For this review, use the dimensioned drawing (mm, ordinates from the lowest corner) and the shaded views. A direction names the side the tool comes from. Coordinates: 2 decimals unless noted, no trailing zeros. Loops run counter-clockwise (first coordinate to the right, second up) from the corner with the lowest first, then second, coordinate; pieces in that order, holes last. Notation, with made-up numbers: (-13, -31) - (30, -31) arc R31 ccw to (30, -4) - close; hole circle Ø2 at (-7.75, 10.5). An arc over 180 degrees is marked (long way). Answer in a Markdown table with one row per item. Add a question column.
(1) The part is to be moulded in two halves that separate along X. For the marked faces 4, 5 and 6, say which applies: released by +X, released by -X, zero draft, split by the parting line, or undercut.
(2) For the marked faces 1, 2 and 3, list the 3-axis set-ups (+Z, -Z, +X, -X, +Y, -Y) from which the entire face can be reached by the end or side of a thin tool; tool diameter is ignored.
(3) Clearance check with flat-ended pins moving along their axes: pin 1 (5 mm diameter, centred on x = 12.5, y = 2, fed in from -Z); pin 2 (6 mm diameter, centred on x = 7, y = 3, fed in from +Z). State where each tip first meets the part, or that it passes through.
(4) We need section A-A, the plane z = 102. Write out the cut boundary in (x, y), plus the area to 3 significant figures.
(5) To check wall thickness, follow L1, parallel to X at y = 9.25, z = 40; L2, parallel to Z at x = 9.75, y = 9.5; L3, parallel to Z at x = 17.5, y = 8.75. State the ranges of each line that lie inside material, in increasing order. Write a range as [from, to].
(6) We need section C-C, the plane x = 13.5. Write out the cut boundary in (y, z), plus the area to 3 significant figures.
(7) We need section B-B, the plane y = 10.5. Write out the cut boundary in (x, z).
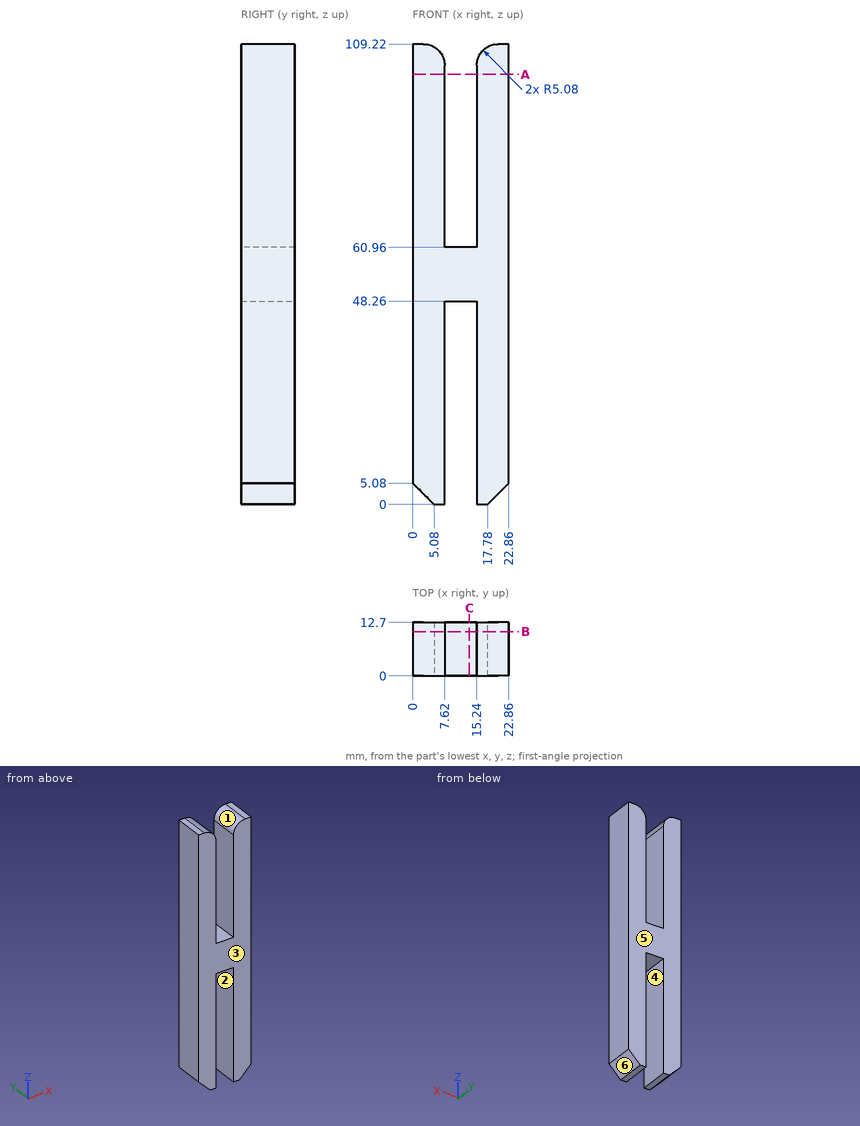
Responses:
| question | item | result |
|---|---|---|
| 1 | face 4 | undercut |
| 1 | face 5 | zero draft |
| 1 | face 6 | released by +X |
| 2 | face 1 | +Z, +Y, -Y |
| 2 | face 2 | -Z, +Y, -Y |
| 2 | face 3 | +Z, -Z, +X, -X, -Y |
| 3 | pin 1 | stops at z = 48.26 |
| 3 | pin 2 | stops at z = 109.01 |
| 4 | outline | (0, 0) - (7.62, 0) - (7.62, 12.7) - (0, 12.7) - close; (15.24, 0) - (22.86, 0) - (22.86, 12.7) - (15.24, 12.7) - close |
| 4 | area | 194 mm2 |
| 5 | L1 | x = [0, 7.62], [15.24, 22.86] |
| 5 | L2 | z = [48.26, 60.96] |
| 5 | L3 | z = [0, 108.37] |
| 6 | outline | (0, 48.26) - (12.7, 48.26) - (12.7, 60.96) - (0, 60.96) - close |
| 6 | area | 161 mm2 |
| 7 | outline | (0, 5.08) - (5.08, 0) - (7.62, 0) - (7.62, 48.26) - (15.24, 48.26) - (15.24, 0) - (17.78, 0) - (22.86, 5.08) - (22.86, 109.22) - (20.32, 109.22) arc R5.08 ccw to (15.24, 104.14) - (15.24, 60.96) - (7.62, 60.96) - (7.62, 104.14) arc R5.08 ccw to (2.54, 109.22) - (0, 109.22) - close |
